The listing builds one solid part. Answer for the finished solid, in the listing's coordinates (mm). Give positions to 0.01 mm unless a question says otherwise; leave off trailing zeros. Loops run counter-clockwise (first coordinate to the right, second up) from the corner with the lowest first, then second, coordinate; pieces in that order, holes last.
Item 1: Consider line 1 along Y through (x, z) = (-5, 33); line 2 along Y through (x, z) = (-6.5, 8); line 3 along Y through (x, z) = (-8.75, 8.5). Determine where each line is inside the solid, lowest interval first.
Item 2: This flat-tipped pin is pushed along its axis until it touches: pin 1 Ø3.5 at (x, y) = (5, -19) entering from +Z. Where does it stop, or does it pass through?
Item 3: Section A-A, the plane z = 29.5 is taken. Give the vertices of the cut face in (x, y).
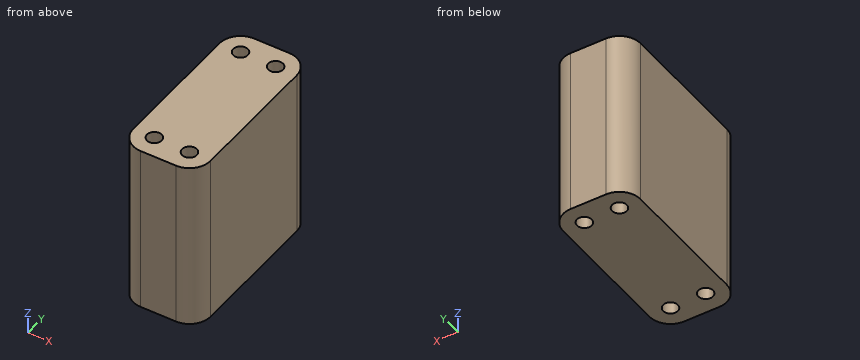
from build123d import *

# Parameters (mm, degrees)
ESQUISSE1_W             = 22
ESQUISSE1_H             = 50
BOSS_EXTRU_1_DEPTH      = 48.514
CONG_1_R                = 6
ESQUISSE2_R             = 2.1
ENL_V_MAT_EXTRU_1_DEPTH = 56.674125013


with BuildPart() as part:
    # Esquisse1 → Boss.-Extru.1 (new body)
    with BuildSketch(Plane.XY):
        Rectangle(ESQUISSE1_W, ESQUISSE1_H)
    extrude(amount=BOSS_EXTRU_1_DEPTH)

    # Congé1
    cong_1_edges = [part.edges().sort_by_distance(p)[0] for p in [
        (-11, 25, 24.257),
        (11, 25, 24.257),
        (11, -25, 24.257),
        (-11, -25, 24.257),
    ]]
    fillet(cong_1_edges, radius=CONG_1_R)

    # Esquisse2 → Enlèv. mat.-Extru.1 (cut, through all)
    with BuildSketch(Plane.XY.offset(48.514)):
        with Locations((-5, 19)):
            Circle(ESQUISSE2_R)
        with Locations((5, 19)):
            Circle(ESQUISSE2_R)
        with Locations((-5, -19)):
            Circle(ESQUISSE2_R)
        with Locations((5, -19)):
            Circle(ESQUISSE2_R)
    extrude(amount=-ENL_V_MAT_EXTRU_1_DEPTH, mode=Mode.SUBTRACT)


solid = part.part
Worked answers:
1. line 1: y = -25 to -21.1, -16.9 to 16.9, 21.1 to 25
1. line 2: y = -24.81 to -20.47, -17.53 to 17.53, 20.47 to 24.81
1. line 3: y = -23.68 to 23.68
2. pin 1: passes through
3. outline: (-11, -19) arc R6 ccw to (-5, -25) - (5, -25) arc R6 ccw to (11, -19) - (11, 19) arc R6 ccw to (5, 25) - (-5, 25) arc R6 ccw to (-11, 19) - close; hole circle Ø4.2 at (-5, -19); hole circle Ø4.2 at (-5, 19); hole circle Ø4.2 at (5, -19); hole circle Ø4.2 at (5, 19)
